from build123d import *

# Parameters (mm, degrees)
SKETCH2_R           = 4.975
BOSS_EXTRUDE1_DEPTH = 5
SKETCH3_R           = 5.97
BOSS_EXTRUDE2_DEPTH = 5
SKETCH5_R           = 5.97
BOSS_EXTRUDE3_DEPTH = 5
SKETCH6_R           = 4.975
BOSS_EXTRUDE4_DEPTH = 5
SKETCH8_R           = 2.698107805
BOSS_EXTRUDE5_DEPTH = 4.6
CUT_EXTRUDE3_DEPTH  = 16.1
SKETCH12_R          = 2.646
CUT_EXTRUDE4_DEPTH  = 3
CUT_EXTRUDE5_DEPTH  = 1.5


with BuildPart() as part:
    # Sketch2 → Boss-Extrude1 (new body)
    with BuildSketch(Plane.XY.offset(10.054948089)):
        Circle(SKETCH2_R)
        with BuildLine():
            Line((2, 1.5), (2, -1.5))
            ThreePointArc((2, -1.5), (-2.5, 0), (2, 1.5))
        make_face(mode=Mode.SUBTRACT)
    extrude(amount=BOSS_EXTRUDE1_DEPTH)

    # Sketch3 → Boss-Extrude2 (add)
    with BuildSketch(Plane.XY.offset(15.054948089)):
        with Locations((0.75, 0)):
            Circle(SKETCH3_R)
        with BuildLine():
            Line((2, 1.5), (2, -1.5))
            ThreePointArc((2, -1.5), (-2.5, -1e-09), (2, 1.5))
        make_face(mode=Mode.SUBTRACT)
    extrude(amount=BOSS_EXTRUDE2_DEPTH)

    # Sketch5 → Boss-Extrude3 (add)
    with BuildSketch(Plane.XY.offset(20.054948089)):
        with Locations(Location((-0.75, 0, 0), (0, 0, 277.217031551))):
            Circle(SKETCH5_R)
        with BuildLine():
            Line((2, 1.5), (2, -1.5))
            ThreePointArc((2, -1.5), (-2.5, 0), (2, 1.5))
        make_face(mode=Mode.SUBTRACT)
    extrude(amount=BOSS_EXTRUDE3_DEPTH)

    # Sketch6 → Boss-Extrude4 (add)
    with BuildSketch(Plane.XY.offset(25.054948089)):
        Circle(SKETCH6_R)
        with BuildLine():
            Line((2, 1.5), (2, -1.5))
            ThreePointArc((2, -1.5), (-2.5, 0), (2, 1.5))
        make_face(mode=Mode.SUBTRACT)
    extrude(amount=BOSS_EXTRUDE4_DEPTH)

    # Sketch8 → Boss-Extrude5 (add)
    with BuildSketch(Plane.XY.offset(25.454948089)):
        Circle(SKETCH8_R)
    extrude(amount=BOSS_EXTRUDE5_DEPTH)

    # Sketch10 → Cut-Extrude3 (cut)
    with BuildSketch(Plane(origin=(0, 0, 10.054948089), x_dir=(-1, 0, 0), z_dir=(0, 0, -1))):
        with BuildLine():
            Line((-2.127176471, 1.57366968), (-2.127176471, -1.57366968))
            ThreePointArc((-2.127176471, -1.57366968), (2.646, 0), (-2.127176471, 1.57366968))
        make_face()
    extrude(amount=-CUT_EXTRUDE3_DEPTH, mode=Mode.SUBTRACT)

    # Sketch12 → Cut-Extrude4 (cut)
    with BuildSketch(Plane(origin=(0, 0, 10.054948089), x_dir=(-1, 0, 0), z_dir=(0, 0, -1))):
        Circle(SKETCH12_R)
    extrude(amount=-CUT_EXTRUDE4_DEPTH, mode=Mode.SUBTRACT)

    # Sketch13 → Cut-Extrude5 (cut)
    with BuildSketch(Plane.XY.offset(30.054948089)):
        with BuildLine():
            ThreePointArc((-2.51116552, -0.087954636), (-1.357302284, 1.973549468), (1.004944259, 1.942072291))
            add(Edge.make_bspline(
                [(1.004944259, 1.942072291), (1.080556299, 1.886286139), (1.19790515, 1.808024326), (1.373021318, 1.656234404), (1.47030803, 1.558406007), (1.550477263, 1.513006562)],
                knots=[0, 0, 0, 0, 0.406231217, 0.607035645, 1, 1, 1, 1], degree=3))
            add(Edge.make_bspline(
                [(1.550477263, 1.513006562), (1.635864774, 1.474239987), (1.773010843, 1.366273459), (2.039141531, 1.334356693), (2.331882187, 1.388131663), (2.66672311, 1.446751803), (2.982241637, 1.541137483), (3.279025568, 1.591865164), (3.523767348, 1.639570409), (3.784019221, 1.657387797), (3.969776334, 1.659661053), (4.168941475, 1.644062658), (4.202381272, 1.52843867), (4.126318671, 1.44725911), (4.010429706, 1.335902318), (3.968265182, 1.291154175), (3.792262006, 1.168081192)],
                knots=[0, 0, 0, 0, 0.086753896, 0.154448198, 0.238460485, 0.359650414, 0.46636505, 0.540243649, 0.635674639, 0.69606208, 0.776341506, 0.817536165, 0.854232706, 0.891997853, 0.906574583, 1, 1, 1, 1], degree=3))
            add(Edge.make_bspline(
                [(2.091354428, -0.087954636), (2.926147793, 0.575225687), (3.792262006, 1.168081192)],
                knots=[0, 0, 0, 1, 1, 1], degree=2))
            ThreePointArc((2.091354428, -0.087954636), (0.943093758, -2.009095653), (-1.294793502, -2.042948055))
            add(Edge.make_bspline(
                [(-1.294793502, -2.042948055), (-1.746909796, -1.848672711), (-1.711703775, -1.762613123), (-1.117517562, -1.523273653)],
                knots=[0, 0, 0, 0, 1, 1, 1, 1], degree=3))
            add(Edge.make_bspline(
                [(-1.117517562, -1.523273653), (-0.851635042, -1.433760086), (-0.637638887, -1.542714277)],
                knots=[0, 0, 0, 1, 1, 1], degree=2))
            ThreePointArc((-0.637638887, -1.542714277), (0.768418454, -1.247154446), (1.362404266, 0.061101538))
            add(Edge.make_bspline(
                [(1.362404266, 0.061101538), (1.355019388, 0.205736583), (1.311882289, 0.343336372)],
                knots=[0, 0, 0, 1, 1, 1], degree=2))
            add(Edge.make_bspline(
                [(1.311882289, 0.343336372), (1.271394274, 0.321666217), (0.98055525, 0.164223835), (0.484149511, -0.131008667), (-0.185861153, -0.47298164), (-0.847852238, -0.872955403), (-1.568325935, -1.264471006), (-2.337842685, -1.536065016), (-3.003283347, -1.787232277), (-3.502067412, -1.898250422), (-3.821928849, -1.960496005), (-4.017644788, -1.891018555), (-3.987917105, -1.67782918), (-3.819171551, -1.496110904), (-3.60958725, -1.238739607), (-3.341385255, -0.983372917), (-3.09159848, -0.713615899), (-2.794092314, -0.437511254), (-2.628823727, -0.204972872), (-2.51116552, -0.087954636)],
                knots=[0.23960858, 0.23960858, 0.23960858, 0.23960858, 0.252432001, 0.331936596, 0.400251659, 0.461905574, 0.547436375, 0.628008605, 0.68882094, 0.745646596, 0.769268725, 0.780800749, 0.795535828, 0.817809693, 0.851462573, 0.887178783, 0.921045432, 0.953843573, 1, 1, 1, 1], degree=3))
        make_face()
        with BuildLine():
            ThreePointArc((1.157395644, 0.783657031), (-0.928142572, 1.617548229), (-1.712921676, -0.486962626))
            add(Edge.make_bspline(
                [(-1.712921676, -0.486962626), (-1.384473336, -0.532536822), (-0.992466447, -0.411621309), (-0.517874245, -0.15891637)],
                knots=[0, 0, 0, 0, 1, 1, 1, 1], degree=3))
            add(Edge.make_bspline(
                [(-0.517874245, -0.15891637), (0.320919337, 0.310316941), (1.157395644, 0.783657031)],
                knots=[0, 0, 0, 1, 1, 1], degree=2))
        make_face(mode=Mode.SUBTRACT)
    extrude(amount=-CUT_EXTRUDE5_DEPTH, mode=Mode.SUBTRACT)


solid = part.part
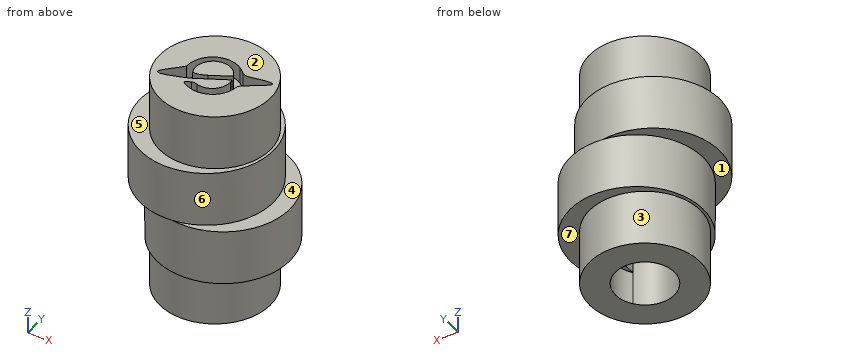
Geometry check sheet. Reference: the model listing, model coordinates, mm. Face numbers are marked on the shaded views. A direction names the side the tool comes from. Give positions to 0.01 mm unless a question says otherwise; leave off trailing zeros. Write each loop counter-clockwise with the first axis right and the second up, starting at its lowest first coordinate (ties: lowest second). Pieces come first, ordered by that corner, then holes.
1) Go/stop test with flat-tipped pins: pin 1 Ø3 at (y, z) = (3.5, 18) entering from -X (3 decimals); pin 2 Ø3.5 at (y, z) = (-1, 18) entering from -X; pin 3 Ø5 at (x, z) = (-5, 18.5) entering from +Y. Record where each tip stops, or that it passes through.
Values follow:
pin 1: stops at x = -4.875
pin 2: stops at x = -5.22
pin 3: stops at y = 5.51
2) Set-up check for the marked faces 1, 2, 3, 4 and 5: record each of +Z, -Z, +X, -X, +Y, -Y from which the full face is reachable in a straight line by a thin tool's end or side.
Values follow:
face 1: -Z, -X
face 2: +Z, +X, -X, +Y, -Y
face 3: -Z
face 4: +Z, +X
face 5: +Z
3) Thickness scan on line 1 (X direction, y = 0, z = 19.75); line 2 (Y direction, x = 0, z = 14.5) (3 decimals); line 3 (X direction, y = 0, z = 21.5). Record the ranges inside material, lowest first.
Values follow:
line 1: x = -5.22 to -2.65, 2.13 to 6.72
line 2: y = -4.975 to -2.646, 2.646 to 4.975
line 3: x = -6.72 to -2.65, 2.13 to 5.22
4) Cross-section at D-D (z = 19.75). Record the boundary of the cut face in (x, y).
Values follow:
outline: circle Ø11.94 at (0.75, 0); hole (2.13, -1.57) - (2.13, 1.57) arc R2.65 ccw (long way) to start
5) Cross-section at C-C (x = -5.5). Record the boundary of the cut face in (y, z).
Values follow:
outline: (-3.62, 20.05) - (3.62, 20.05) - (3.62, 25.05) - (-3.62, 25.05) - close
6) Cross-section at A-A (z = 12.5). Record the boundary of the cut face in (x, y) (3 decimals), plus the area to 3 significant figures.
Values follow:
outline: circle Ø9.95 at (0, 0); hole circle Ø5.292 at (0, 0)
area: 55.8 mm2
7) Release check for a two-part mould opening along Y. For the marked faces 6 and 7 record: released by +Y, released by -Y, zero draft, split by the parting line, or undercut.
Values follow:
face 6: split by the parting line
face 7: zero draft
8) Cross-section at B-B (y = -4.25). Record the boundary of the cut face in (x, z), plus the area to 3 significant figures.
Values follow:
outline: (-4.94, 20.05) - (-3.44, 20.05) - (-3.44, 15.05) - (-2.59, 15.05) - (-2.59, 10.05) - (2.59, 10.05) - (2.59, 15.05) - (4.94, 15.05) - (4.94, 20.05) - (3.44, 20.05) - (3.44, 25.05) - (2.59, 25.05) - (2.59, 30.05) - (-2.59, 30.05) - (-2.59, 25.05) - (-4.94, 25.05) - close
area: 136 mm2
